```python
from build123d import *

# Parameters (mm, degrees)
BOSS_EXTRUDE1_DEPTH = 2
BOSS_EXTRUDE2_DEPTH = 2
SKETCH3_R           = 2.5
CUT_EXTRUDE1_DEPTH  = 10
FILLET1_R           = 1


with BuildPart() as part:
    # Sketch1 → Boss-Extrude1 (new body)
    with BuildSketch(Plane.XY):
        with BuildLine():
            Line((36.5, -14.5), (-36.5, -14.5))
            ThreePointArc((-36.5, -14.5), (-37.914213562, -13.914213562), (-38.5, -12.5))
            Line((-38.5, -12.5), (-38.5, 12.5))
            ThreePointArc((-38.5, 12.5), (-37.914213562, 13.914213562), (-36.5, 14.5))
            Line((-36.5, 14.5), (36.5, 14.5))
            ThreePointArc((36.5, 14.5), (37.914213562, 13.914213562), (38.5, 12.5))
            Line((38.5, 12.5), (38.5, -12.5))
            ThreePointArc((38.5, -12.5), (37.914213562, -13.914213562), (36.5, -14.5))
        make_face()
    extrude(amount=BOSS_EXTRUDE1_DEPTH)

    # Sketch2 → Boss-Extrude2 (add)
    with BuildSketch(Plane.XY.offset(2)):
        with BuildLine():
            Line((34.5, -12.5), (-34.5, -12.5))
            ThreePointArc((-34.5, -12.5), (-35.914213562, -11.914213562), (-36.5, -10.5))
            Line((-36.5, -10.5), (-36.5, 10.5))
            ThreePointArc((-36.5, 10.5), (-35.914213562, 11.914213562), (-34.5, 12.5))
            Line((-34.5, 12.5), (34.5, 12.5))
            ThreePointArc((34.5, 12.5), (35.914213562, 11.914213562), (36.5, 10.5))
            Line((36.5, 10.5), (36.5, -10.5))
            ThreePointArc((36.5, -10.5), (35.914213562, -11.914213562), (34.5, -12.5))
        make_face()
    extrude(amount=BOSS_EXTRUDE2_DEPTH)

    # Sketch3 → Cut-Extrude1 (cut)
    with BuildSketch(Plane(origin=(0, 0, 0), x_dir=(-1, 0, 0), z_dir=(0, 0, -1))):
        with Locations((-30.450412323, -5.952241092)):
            Circle(SKETCH3_R)
        with Locations((-20.450412323, -5.952241092)):
            Circle(SKETCH3_R)
    extrude(amount=-CUT_EXTRUDE1_DEPTH, mode=Mode.SUBTRACT)

    # Fillet1
    fillet1_edges = [part.edges().sort_by_distance(p)[0] for p in [
        (38.5, 0, 0),
        (37.914213562, -13.914213562, 0),
        (0, -14.5, 0),
        (-37.914213562, -13.914213562, 0),
        (-38.5, 0, 0),
        (-37.914213562, 13.914213562, 0),
        (0, 14.5, 0),
        (37.914213562, 13.914213562, 0),
    ]]
    fillet(fillet1_edges, radius=FILLET1_R)


solid = part.part
```
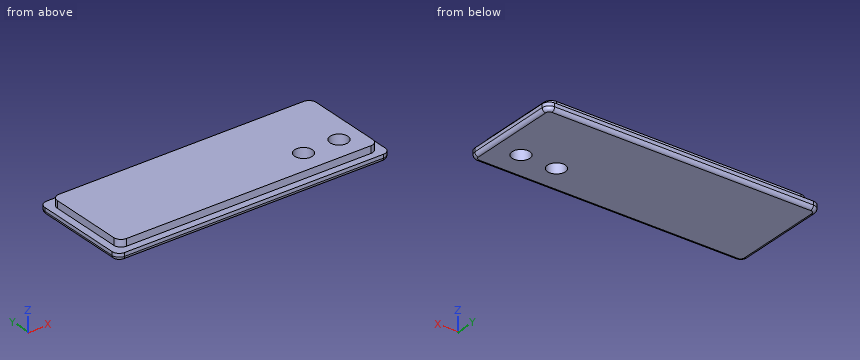
CAD build for the part. Positions are in the model's coordinates, mm. Coordinates: 2 decimals unless noted, no trailing zeros. Loops run counter-clockwise (first coordinate to the right, second up) from the corner with the lowest first, then second, coordinate; pieces in that order, holes last. Notation, with made-up numbers: (63, -28) - (68, -28) arc R28 ccw to (68, 9) - close; hole circle Ø5 at (89, 60.25). An arc over 180 degrees is marked (long way). Return JSON: item names as keys, results as strings.
1. Band-saw the part on D-D (z = 2.9). Give the cut face in (x, y).
Result:
{"outline": "(-36.5, -10.5) arc R2 ccw to (-34.5, -12.5) - (34.5, -12.5) arc R2 ccw to (36.5, -10.5) - (36.5, 10.5) arc R2 ccw to (34.5, 12.5) - (-34.5, 12.5) arc R2 ccw to (-36.5, 10.5) - close; hole circle Ø5 at (20.45, -5.95); hole circle Ø5 at (30.45, -5.95)"}
2. Drop flat-ended pins along their axis: pin 1 (0.6 mm diameter, centred on y = -5, z = 3, fed in from +X); pin 2 (2 mm diameter, centred on y = 8, z = 3.5, fed in from -X). Give the stop position or say it passes through.
Result:
{"pin 1": "stops at x = 36.5", "pin 2": "stops at x = -36.5"}
3. Band-saw the part on B-B (y = -7). Give the cut face in (x, z), and give its area (3 significant figures).
Result:
{"outline": "(-38.5, 1) arc R1 ccw to (-37.5, 0) - (18.18, 0) - (18.18, 4) - (-36.5, 4) - (-36.5, 2) - (-38.5, 2) - close; (22.72, 0) - (28.18, 0) - (28.18, 4) - (22.72, 4) - close; (32.72, 0) - (37.5, 0) arc R1 ccw to (38.5, 1) - (38.5, 2) - (36.5, 2) - (36.5, 4) - (32.72, 4) - close", "area": "263 mm2"}
4. Band-saw the part on A-A (x = 21). Give the cut face in (y, z).
Result:
{"outline": "(-14.5, 1) arc R1 ccw to (-13.5, 0) - (-8.39, 0) - (-8.39, 4) - (-12.5, 4) - (-12.5, 2) - (-14.5, 2) - close; (-3.51, 0) - (13.5, 0) arc R1 ccw to (14.5, 1) - (14.5, 2) - (12.5, 2) - (12.5, 4) - (-3.51, 4) - close"}
5. Band-saw the part on C-C (x = 1). Give the cut face in (y, z).
Result:
{"outline": "(-14.5, 1) arc R1 ccw to (-13.5, 0) - (13.5, 0) arc R1 ccw to (14.5, 1) - (14.5, 2) - (12.5, 2) - (12.5, 4) - (-12.5, 4) - (-12.5, 2) - (-14.5, 2) - close"}
6. Probe L1, parallel to X at y = -7.25, z = 1; L2, parallel to X at y = -6.75, z = 1.9; L3, parallel to Y at x = -33, z = 2.1. List the from-to ranges inside material, lowest first. Write a range as from..to.
Result:
{"L1": "x = -38.5..18.31, 22.59..28.31, 32.59..38.5", "L2": "x = -38.5..18.08, 22.82..28.08, 32.82..38.5", "L3": "y = -12.5..12.5"}
